Geometry: final body of the model. Coordinates: model frame, mm. Face numbers are marked on the shaded views. A direction names the side the tool comes from. Give positions to 0.01 mm unless a question says otherwise; leave off trailing zeros. Write each loop counter-clockwise with the first axis right and the second up, starting at its lowest first coordinate (ties: lowest second). Pieces come first, ordered by that corner, then holes.
Q1. Cut plane D-D on y = 19. Return the cut outline in (x, z).
Q2. Pin query (flat end, axial travel): pin 1 (7.5 mm diameter, centred on x = 1, y = 20, fed in from +Z); pin 2 (3 mm diameter, centred on x = 0, z = 15, fed in from +Y); pin 3 (1 mm diameter, centred on x = 1.5, z = 16, fed in from -Y); pin 4 (2.5 mm diameter, centred on x = 0, y = -19, fed in from -Z). Return the tip coordinate at first contact, or that it passes through.
Q3. Draft query along Y for the marked faces 1, 2, 3 and 4. Return one class per face: pulls with the +Y half, pulls with the -Y half, needs draft (parallel to the pull), parting line crosses it, or undercut.
Q4. Cut plane B-B on z = 15. Return the cut outline in (x, y), plus the area to 3 significant figures.
Q5. Cut plane C-C on x = -9. Return the cut outline in (y, z), plus the area to 3 significant figures.
Q6. Line query: L1, parallel to Y at x = 0, z = 2.25; L2, parallel to Z at x = 0, y = 5.5; L3, parallel to Y at x = 14, z = 6.25. Output: solid intervals per line, ascending.
Q7. Reachability of the marked faces 5, 6 and 7 from +Z, -Z, +X, -X, +Y, -Y: full face, straight path, thin tool, end or side. Return the list, or none.
Q8. Cut plane A-A on y = 4.5. Return the cut outline in (x, z).
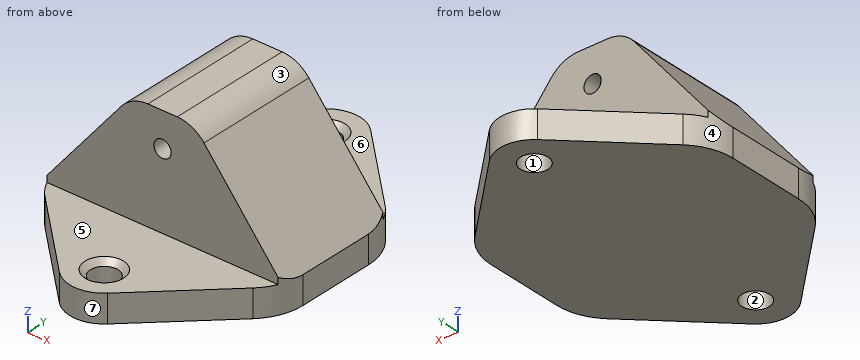
Autodesk Inventor part; units mm, degrees
ref_plane "YZ Plane" through (0, 0, 0) normal (1, 0, 0) x (0, 1, 0)
ref_plane "XZ Plane" through (0, 0, 0) normal (0, 1, 0) x (-1, 0, 0)
ref_plane "XY Plane" through (0, 0, 0) normal (0, 0, 1) x (1, 0, 0)
sketch "Sketch1" plane through (0, 0, 0) normal (0, 0, 1) x (1, 0, 0)
  line L0 (-17.5, 9) -> (17.5, 9)
  line L1 (17.5, 9) -> (17.5, -9)
  line L2 (17.5, -9) -> (-17.5, -9)
  line L3 (-17.5, -9) -> (-17.5, 9)
  circle A0 centre (0, 19) radius 5
  line L4 (-17.5, 9) -> (-3.4801, 22.5901)
  line L5 (17.5, 9) -> (3.4801, 22.5901)
  circle A1 centre (0, 19) radius 2
  point P0 (0, 0)
  dimension "d0" = 35
  dimension "d1" = 18
  dimension "d5" = 17.5
  dimension "d6" = 9
  dimension "d13" = 10
  dimension "d14" = 10
  dimension "d15" = 4
extrude "Extrusion1" add sketch "Sketch1" along normal blind 20 contours L0 L1 L2 L3
extrude "Extrusion3" add sketch "Sketch1" along normal blind 4 contours L4 A0 L5 L0 | A0
mirror "Mirror3" about plane through (0, 0, 0) normal (0, 1, 0) of "Extrusion3"
chamfer "Chamfer1" distance 13 distance2 16 1 edges at (17.5, 0, 20) measured on face at (5.8333, -3, 20)
chamfer "Chamfer2" distance 13 distance2 16 1 edges at (-17.5, 0, 20) measured on face at (-10.1667, 3, 20)
sketch "Sketch2" plane through (-17.5, -9, 4) normal (0, -1, 0) x (1, 0, 0)
  line L0 (0, 0) -> (13, 16)
  line L1 (0, 0) -> (35, 0)
  line L2 (22, 16) -> (35, 0)
  line L3 (13, 16) -> (22, 16)
  point P0 (17.5, -4)
  point P1 (17.5, 11)
  dimension "d24" = 35
  dimension "d25" = 17.5
  dimension "d26" = 5
hole "Hole1" at (0, -9, 15) direction (0, 1, 0) diameter 2.5 end through all
fillet "Fillet1" radius 5 2 edges at (-4.5, 0, 20) (4.5, 0, 20)
fillet "Fillet2" radius 8 4 edges at (-17.5, -9, 2) (-17.5, 9, 2) (17.5, -9, 2) (17.5, 9, 2)
chamfer "Chamfer3" distance 0.8 angle 45 2 edges at (-2, -19, 4) (-2, 19, 4)
properties part number "3DP_PLA_Measurement_Rail_Base" material "ABS Plastic"
Data:
1. outline: (-7.18, 0) - (-2, 0) - (-2, 3.2) - (-2.8, 4) - (-7.18, 4) - close; (2, 0) - (7.18, 0) - (7.18, 4) - (2.8, 4) - (2, 3.2) - close
2. pin 1: stops at z = 4
2. pin 2: stops at y = 9
2. pin 3: stops at y = -9
2. pin 4: passes through
3. face 1: undercut
3. face 2: undercut
3. face 3: needs draft
3. face 4: pulls with the +Y half
4. outline: (-8.56, -9) - (-1.25, -9) - (-1.25, 9) - (-8.56, 9) - close; (1.25, -9) - (8.56, -9) - (8.56, 9) - (1.25, 9) - close
4. area: 263 mm2
5. outline: (-17.24, 0) - (17.24, 0) - (17.24, 4) - (9, 4) - (9, 14.46) - (-9, 14.46) - (-9, 4) - (-17.24, 4) - close
5. area: 326 mm2
6. L1: y = -24 to -21, -17 to 17, 21 to 24
6. L2: z = 0 to 13.75, 16.25 to 20
6. L3: y = -9 to 9
7. face 5: +Z, +X, -X, -Y
7. face 6: +Z, +X, -X, +Y
7. face 7: +Z, -Z, -Y
8. outline: (-17.5, 0) - (17.5, 0) - (17.5, 4) - (6, 18.15) arc R5 ccw to (2.12, 20) - (-2.12, 20) arc R5 ccw to (-6, 18.15) - (-17.5, 4) - close; hole circle Ø2.5 at (0, 15)
